Could you check a few things on this model? Use its own coordinates, in mm. A direction names the side the tool comes from. Round coordinates to 2 decimals unless told otherwise and drop trailing zeros. Loops run counter-clockwise (first coordinate to the right, second up) from the corner with the lowest first, then second, coordinate; pieces in that order, holes last.
from build123d import *

# Parameters (mm, degrees)
SKETCH1_R               = 30.595
BOSS_EXTRUDE1_DEPTH     = 90
BOSS_EXTRUDE1_DRAFT     = -12
SKETCH2_R               = 15
CUT_EXTRUDE1_DEPTH      = 50
CUT_EXTRUDE4_DEPTH      = 115.215451058
CUT_EXTRUDE4_DEPTH_BACK = 115.215451058
SKETCH3_R               = 15


with BuildPart() as part:
    # Sketch1 → Boss-Extrude1 (with draft: the straight prism first)
    with BuildSketch(Plane.XY):
        Circle(SKETCH1_R)
    extrude(amount=BOSS_EXTRUDE1_DEPTH)
    # Boss-Extrude1: the draft: its side faces are tilted about the plane it starts from
    boss_extrude1_sides = [part.faces().sort_by_distance(p)[0] for p in [
        (-30.595, 0, 45),
    ]]
    draft(boss_extrude1_sides, Plane.XY, BOSS_EXTRUDE1_DRAFT)

    # Sketch2 → Cut-Extrude1 (cut)
    with BuildSketch(Plane(origin=(0, 0, 0), x_dir=(-1, 0, 0), z_dir=(0, 0, -1))):
        Circle(SKETCH2_R)
    extrude(amount=-CUT_EXTRUDE1_DEPTH, mode=Mode.SUBTRACT)

    # Sketch3 → Cut-Extrude4 (cut, two sides: drawn at the far end of the back side and taken through both)
    with BuildSketch(Plane(origin=(0, 0, 0), x_dir=(0, 0, -1), z_dir=(1, 0, 0)).offset(-CUT_EXTRUDE4_DEPTH_BACK)):
        with Locations((-90, 0)):
            Circle(SKETCH3_R)
    extrude(amount=CUT_EXTRUDE4_DEPTH + CUT_EXTRUDE4_DEPTH_BACK, mode=Mode.SUBTRACT)


solid = part.part
Item 1: If we section it at B-B, the plane z = 79: Please give me the cut outline in (x, y).
Results list:
outline: (-46.28, -10.2) arc R47.39 ccw to (46.28, -10.2) - close; (-46.28, 10.2) - (46.28, 10.2) arc R47.39 ccw to start
Item 2: Will these pins go through, and if not, where does the flat tip stop? pin 1 (2 mm diameter, centred on x = -17, z = 42, fed in from -Y); pin 2 (12 mm diameter, centred on x = -17.5, z = 61.5, fed in from -Y); pin 3 (8 mm diameter, centred on y = 22.5, z = 31, fed in from +X).
Results list:
pin 1: stops at y = -36.2
pin 2: stops at y = -42.58
pin 3: stops at x = 32.46
Item 3: If I drill on line 1 along Y through (x, z) = (-29.5, 79.5); line 2 along X through (y, z) = (-13, 15); line 3 along X through (y, z) = (-3, 54), over which ranges is the centre line in solid material (lowest first)?
Results list:
line 1: y = -37.22 to -10.71, 10.71 to 37.22
line 2: x = -31.18 to -7.48, 7.48 to 31.18
line 3: x = -41.97 to 41.97
Item 4: If we section it at C-C, the plane y = 0: Please give me the cut outline in (x, z) (3 decimals), then the cut area to 3 significant figures.
Results list:
outline: (-46.537, 75) - (-30.595, 0) - (-15, 0) - (-15, 50) - (15, 50) - (15, 0) - (30.595, 0) - (46.537, 75) - close
area: 4,280 mm2
Item 5: For faces 1 (the flat face through (-1, -28, 90)), 2 (the cylindrical face through (14.985, 0.66, 24.65)), which set-ups out of +Z, -Z, +X, -X, +Y, -Y let a thin tool reach every point of the face, with its end or its side?
Results list:
face 1: +Z, +X, -X, +Y, -Y
face 2: -Z
Item 6: We'd pull the mould along Y, two halves only. Please class faces 3 (the conical face through (36.15, 11.38, 34.37)), 4 (the flat face through (-14, -6, 0)), 5 (the cylindrical face through (-1, 0, 75)): released by +Y, released by -Y, zero draft, split by the parting line, or undercut.
Results list:
face 3: split by the parting line
face 4: zero draft
face 5: undercut
Item 7: If we section it at A-A, the plane x = 0: Please give me the cut outline in (y, z) (3 decimals).
Results list:
outline: (-49.725, 90) - (-30.595, 0) - (-15, 0) - (-15, 50) - (15, 50) - (15, 0) - (30.595, 0) - (49.725, 90) - (15, 90) arc R15 cw to (-15, 90) - close
Item 8: If we section it at D-D, the plane z = 41.5: Please give me the cut outline in (x, y), then the cut area to 3 significant figures.
Results list:
outline: circle Ø78.83 at (0, 0); hole circle Ø30 at (0, 0)
area: 4,170 mm2
